Answer from the drawing. Dimensions are ordinates in mm from the lowest x, y and z of the part. A direction names the side the tool comes from. Give positions to 0.01 mm unless a question says otherwise; leave off trailing zeros. Write each loop counter-clockwise with the first axis right and the second up, starting at its lowest first coordinate (ties: lowest second). Pieces come first, ordered by that corner, then holes. Notation, with made-up numbers: M 10.5,67 L 19.5,67 A5 cw 19.5,73 Z; hole C 21.25,8 d3. An arc over 180 degrees is marked long. Answer as a JSON object with one key per item and string values.
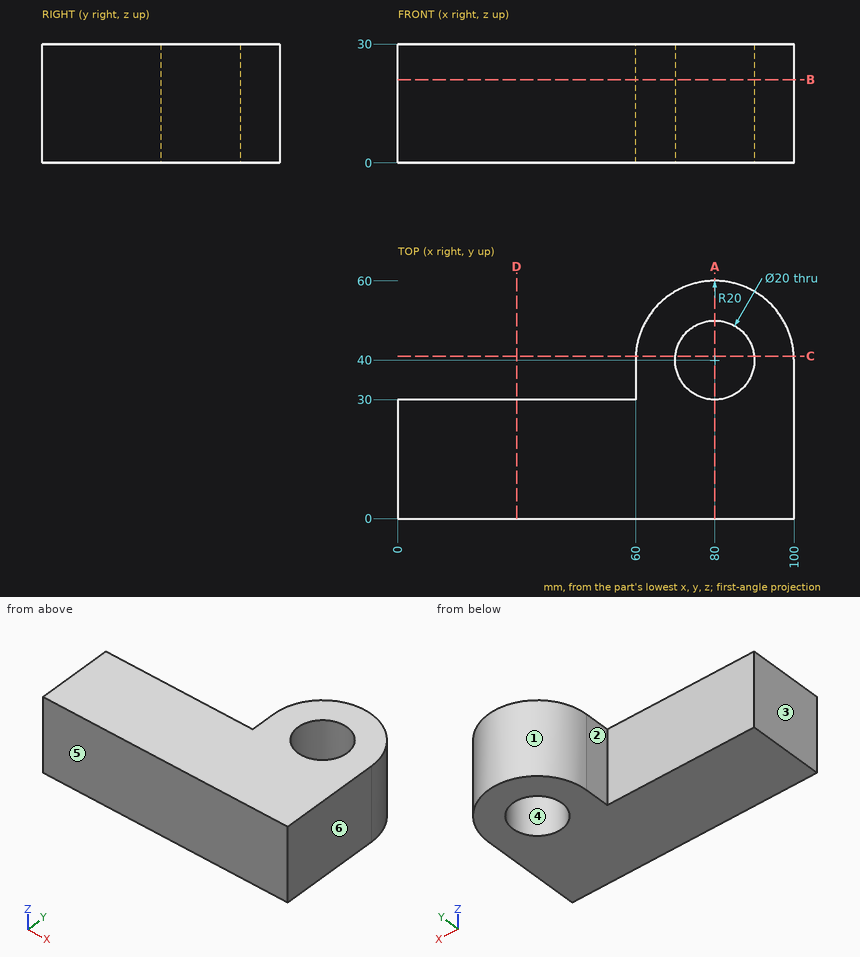
1. The mould has two halves that part along X. Classify the marked faces 3, 4, 5 and 6: released by +X, released by -X, zero draft, split by the parting line, or undercut.
Verdict:
{"face 3": "released by -X", "face 4": "undercut", "face 5": "zero draft", "face 6": "released by +X"}
2. A cutting plane is placed at B-B, the plane z = 21. Give the vertices of the cut face in (x, y), plus the area to 3 significant figures.
Verdict:
{"outline": "M 0,0 L 100,0 L 100,40 A20 ccw 60,40 L 60,30 L 0,30 Z; hole C 80,40 d20", "area": "3,710 mm2"}
3. A cutting plane is placed at C-C, the plane y = 41. Give the vertices of the cut face in (x, z), plus the area to 3 significant figures.
Verdict:
{"outline": "M 60.03,0 L 70.05,0 L 70.05,30 L 60.03,30 Z; M 89.95,0 L 99.97,0 L 99.97,30 L 89.95,30 Z", "area": "602 mm2"}
4. For the marked faces 1 and 2, determine the directions among +Z, -Z, +X, -X, +Y, -Y from which every point of the face is accessible in a straight line to the end or side of a thin tool.
Verdict:
{"face 1": "+Z, -Z, +Y", "face 2": "+Z, -Z, -X, +Y"}
5. Consider line 1 along Y through (x, z) = (80, 18.5); line 2 along X through (y, z) = (40, 6.5); line 3 along Y through (x, z) = (31.5, 9). Determine where each line is inside the solid, lowest interval first.
Verdict:
{"line 1": "y = 0 to 30, 50 to 60", "line 2": "x = 60 to 70, 90 to 100", "line 3": "y = 0 to 30"}
6. A cutting plane is placed at D-D, the plane x = 30. Give the vertices of the cut face in (y, z), plus the area to 3 significant figures.
Verdict:
{"outline": "M 0,0 L 30,0 L 30,30 L 0,30 Z", "area": "900 mm2"}
7. A cutting plane is placed at A-A, the plane x = 80. Give the vertices of the cut face in (y, z).
Verdict:
{"outline": "M 0,0 L 30,0 L 30,30 L 0,30 Z; M 50,0 L 60,0 L 60,30 L 50,30 Z"}
8. Flat-ended cylindrical pins translate along their axes: pin 1 (12 mm diameter, centred on x = 42.5, y = 16, fed in from -Z); pin 2 (1 mm diameter, centred on x = 16.5, z = 25, fed in from +Y); pin 3 (3 mm diameter, centred on y = 35, z = 8.5, fed in from -X). Find the tip coordinate at first contact, or state that the pin passes through.
Verdict:
{"pin 1": "stops at z = 0", "pin 2": "stops at y = 30", "pin 3": "stops at x = 60"}
